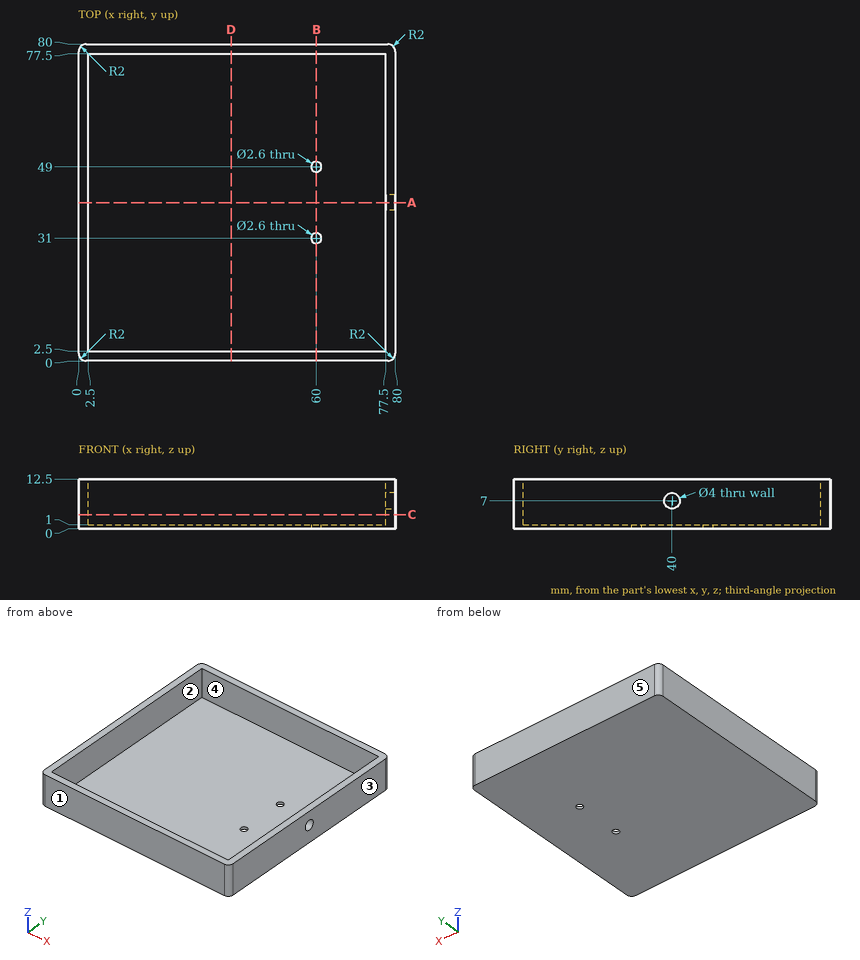
Answer from the drawing. Dimensions are ordinates in mm from the lowest x, y and z of the part. A direction names the side the tool comes from. Round coordinates to 2 decimals unless told otherwise and drop trailing zeros. Write each loop counter-clockwise with the first axis right and the second up, starting at its lowest first coordinate (ties: lowest second). Pieces come first, ordered by that corner, then holes. Notation, with made-up numbers: M 47,85.25 L 87,85.25 A22 cw 87,113.25 Z; hole C 45.5,-17.75 d3. An arc over 180 degrees is marked long. Write each question's results on one line, items separated by ' | '. Start each with the question number.
Item 1: A cutting plane is placed at A-A on y = 40. Write down the section's boundary in (x, z), and give its area (4 significant figures).
Item 2: Straight lines are drawn through the part: L1, parallel to Y at x = 60, z = 0.35; L2, parallel to Y at x = 54.5, z = 6. For each, find the intervals that lie inside material, in ascending order. Write a range as [from, to].
Item 3: For the marked faces 4 and 5, determine the directions among +Z, -Z, +X, -X, +Y, -Y from which every point of the face is accessible in a straight line to the end or side of a thin tool.
Item 4: For a pull along X with two mould halves and no side action, classify the marked faces 1, 2 and 3 as pulls with the +X half, pulls with the -X half, needs draft (parallel to the pull), parting line crosses it, or undercut.
Item 5: A cutting plane is placed at B-B on x = 60. Write down the section's boundary in (y, z).
Item 6: A flat-ended cylindrical pin translates along its axis: pin 1 Ø3 at (y, z) = (40, 7) entering from +X. Find the tip coordinate at first contact, or state that the pin passes through.
Item 7: A cutting plane is placed at C-C on z = 3.5. Write down the section's boundary in (x, y).
Item 8: A cutting plane is placed at D-D on x = 38.5. Write down the section's boundary in (y, z), and give its area (4 significant figures).
Check sheet entries:
1) outline: M 0,0 L 80,0 L 80,5 L 77.5,5 L 77.5,1 L 2.5,1 L 2.5,12.5 L 0,12.5 Z; M 77.5,9 L 80,9 L 80,12.5 L 77.5,12.5 Z | area: 127.5 mm²
2) L1: [0, 29.7], [32.3, 47.7], [50.3, 80] | L2: [0, 2.5], [77.5, 80]
3) face 4: +Z | face 5: +Z, -Z, +X, -X, +Y
4) face 1: needs draft | face 2: undercut | face 3: pulls with the +X half
5) outline: M 0,0 L 29.7,0 L 29.7,1 L 2.5,1 L 2.5,12.5 L 0,12.5 Z; M 32.3,0 L 47.7,0 L 47.7,1 L 32.3,1 Z; M 50.3,0 L 80,0 L 80,12.5 L 77.5,12.5 L 77.5,1 L 50.3,1 Z
6) pin 1: x = 2.5
7) outline: M 0,2 A2 ccw 2,0 L 78,0 A2 ccw 80,2 L 80,78 A2 ccw 78,80 L 2,80 A2 ccw 0,78 Z; hole M 2.5,2.5 L 77.5,2.5 L 77.5,77.5 L 2.5,77.5 Z
8) outline: M 0,0 L 80,0 L 80,12.5 L 77.5,12.5 L 77.5,1 L 2.5,1 L 2.5,12.5 L 0,12.5 Z | area: 137.5 mm²
